Geometry check sheet. Reference: drawing and pictorial views, mm from the part's lowest x, y, z. A direction names the side the tool comes from. Give positions to 0.01 mm unless a question says otherwise; leave off trailing zeros. Order: outer loops, then holes, each group sorted by start corner. A loop starts at its lowest first (then second) coordinate and runs counter-clockwise, first axis right, second up.
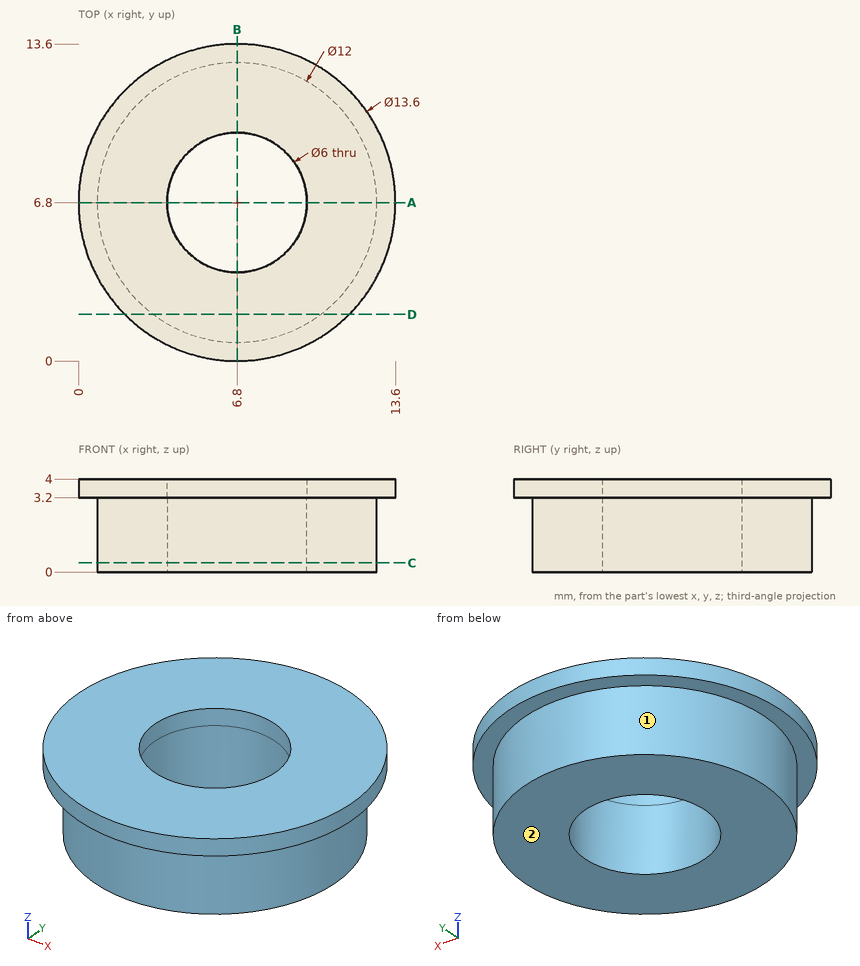
(1) Set-up check for the marked faces 1 and 2: record each of +Z, -Z, +X, -X, +Y, -Y from which the full face is reachable in a straight line by a thin tool's end or side.
Response values:
face 1: -Z
face 2: -Z, +X, -X, +Y, -Y
(2) Cross-section at D-D on y = 2. Enter the section's corners in (x, z).
Response values:
outline: (1.98, 3.2) - (3.2, 3.2) - (3.2, 0) - (10.4, 0) - (10.4, 3.2) - (11.62, 3.2) - (11.62, 4) - (1.98, 4) - close
(3) Gauge pin test, flat end, axial feed: pin 1 Ø2 at (y, z) = (11.5, 1) entering from -X. Record the tip position at first contact, or that the pin passes through.
Response values:
pin 1: stops at x = 2.08
(4) Cross-section at A-A on y = 6.8. Enter the section's corners in (x, z), then the cut area to 3 significant figures.
Response values:
outline: (0, 3.2) - (0.8, 3.2) - (0.8, 0) - (3.8, 0) - (3.8, 4) - (0, 4) - close; (9.8, 0) - (12.8, 0) - (12.8, 3.2) - (13.6, 3.2) - (13.6, 4) - (9.8, 4) - close
area: 25.3 mm2
(5) Cross-section at C-C on z = 0.4. Enter the section's corners in (x, y).
Response values:
outline: circle Ø12 at (6.8, 6.8); hole circle Ø6 at (6.8, 6.8)
(6) Material ranges on L1, parallel to Y at x = 6.8, z = 1.6; L2, parallel to Y at x = 6.8, z = 3.6; L3, parallel to X at y = 9.25, z = 2, recorded low to high.
Response values:
L1: y = 0.8 to 3.8, 9.8 to 12.8
L2: y = 0 to 3.8, 9.8 to 13.6
L3: x = 1.32 to 5.07, 8.53 to 12.28
